Input: part model. Units: mm. Frame: model coordinates. A direction names the side the tool comes from. Coordinates: 2 decimals unless noted, no trailing zeros.
(1) Mould query, pull axis X, two halves, no side actions, for faces 1 (the face through (344, 406, 5)), 2 (the face through (197, 254, 10)). Classes: released by +X, released by -X, zero draft, split by the parting line, or undercut.
(2) Section A-A, the plane z = 2.25. Give the number of separate pieces and of enclosed holes in the cut face, then the cut area to 3 significant figures.
(3) Set-up query: faces 3 (the face through (197, 500, 5)), 4 (the face through (255, 450, 5)), 5 (the face through (369, 414, 5)). Return all of +Z, -Z, +X, -X, +Y, -Y with unobstructed straight access to the full face (end or side cutting, diameter ignored); none if empty.
(4) Line query: L1, parallel to Y at x = 331.75, z = 5.25; L2, parallel to Y at x = 366.5, z = 1; L3, parallel to Y at x = 192.5, z = 3.25. Output: solid intervals per line, ascending.
(5) Contact query for flat-ended pins moving along their axis: P1, Ø5.5, axis at x = 289.5, y = 480, coming from the -Z side; P2, Ø3, axis at y = 362, z = 9, coming from the -X side. Output: stop coordinate, or through.
```python
from build123d import *

# Parameters (mm, degrees)
SKETCH1_W           = 400
SKETCH1_H           = 500
BOSS_EXTRUDE1_DEPTH = 10
CUT_EXTRUDE12_DEPTH = 20
FILLET2_R           = 5
CUT_EXTRUDE16_DEPTH = 32
SKETCH19_R          = 3
SKETCH19_R_2        = 3.35
CUT_EXTRUDE17_DEPTH = 124
CUT_EXTRUDE18_DEPTH = 5


with BuildPart() as part:
    # Sketch1 → Boss-Extrude1 (new body)
    with BuildSketch(Plane.XY):
        with Locations((200, 250)):
            Rectangle(SKETCH1_W, SKETCH1_H)
    extrude(amount=BOSS_EXTRUDE1_DEPTH)

    # Sketch15 → Cut-Extrude12 (cut)
    with BuildSketch(Plane.XY.offset(10)):
        with BuildLine():
            Line((155, 460), (245, 460))
            ThreePointArc((245, 460), (255, 450), (245, 440))
            Line((245, 440), (155, 440))
            ThreePointArc((155, 440), (145, 450), (155, 460))
        make_face()
    extrude(amount=-CUT_EXTRUDE12_DEPTH, mode=Mode.SUBTRACT)

    # Fillet2
    fillet2_edges = [part.edges().sort_by_distance(p)[0] for p in [
        (0, 250, 10),
        (400, 250, 10),
    ]]
    fillet(fillet2_edges, radius=FILLET2_R)

    # Sketch18 → Cut-Extrude16 (cut)
    with BuildSketch(Plane.XY.offset(10)):
        with BuildLine():
            Line((351.5, 399.75), (336.5, 399.75))
            ThreePointArc((336.5, 399.75), (333.75, 402.5), (336.5, 405.25))
            Line((336.5, 405.25), (351.5, 405.25))
            ThreePointArc((351.5, 405.25), (354.25, 402.5), (351.5, 399.75))
        make_face()
        with BuildLine():
            Line((376.5, 407.25), (361.5, 407.25))
            ThreePointArc((361.5, 407.25), (358.75, 410), (361.5, 412.75))
            Line((361.5, 412.75), (376.5, 412.75))
            ThreePointArc((376.5, 412.75), (379.25, 410), (376.5, 407.25))
        make_face()
        with BuildLine():
            Line((376.5, 392.25), (361.5, 392.25))
            ThreePointArc((361.5, 392.25), (358.75, 395), (361.5, 397.75))
            Line((361.5, 397.75), (376.5, 397.75))
            ThreePointArc((376.5, 397.75), (379.25, 395), (376.5, 392.25))
        make_face()
    extrude(amount=-CUT_EXTRUDE16_DEPTH, mode=Mode.SUBTRACT)

    # Sketch19 → Cut-Extrude17 (cut)
    with BuildSketch(Plane(origin=(0, 0, 0), x_dir=(-1, 0, 0), z_dir=(0, 0, -1))):
        with Locations((-380, 145.5)):
            Circle(SKETCH19_R)
        with Locations((-380, 127.5)):
            Circle(SKETCH19_R)
        with Locations((-380, 17)):
            Circle(SKETCH19_R_2)
        with Locations((-17, 17)):
            Circle(SKETCH19_R_2)
        with Locations((-17, 145.5)):
            Circle(SKETCH19_R)
        with Locations((-17, 127.5)):
            Circle(SKETCH19_R)
        with Locations((-113.25, 317.5)):
            Circle(SKETCH19_R)
        with Locations((-113.25, 331.5)):
            Circle(SKETCH19_R)
        with Locations((-151.75, 317.5)):
            Circle(SKETCH19_R)
        with Locations((-151.75, 331.5)):
            Circle(SKETCH19_R)
        with Locations((-293.25, 317.5)):
            Circle(SKETCH19_R)
        with Locations((-293.25, 331.5)):
            Circle(SKETCH19_R)
        with Locations((-331.75, 317.5)):
            Circle(SKETCH19_R)
        with Locations((-331.75, 331.5)):
            Circle(SKETCH19_R)
        with Locations((-17, 336)):
            Circle(SKETCH19_R)
        with Locations((-17, 351)):
            Circle(SKETCH19_R)
        with Locations((-17, 480)):
            Circle(SKETCH19_R_2)
        with Locations((-109.5, 480)):
            Circle(SKETCH19_R)
        with Locations((-127.5, 480)):
            Circle(SKETCH19_R)
        with Locations((-271.5, 480)):
            Circle(SKETCH19_R)
        with Locations((-289.5, 480)):
            Circle(SKETCH19_R)
        with Locations((-380, 480)):
            Circle(SKETCH19_R_2)
        with Locations((-382.5, 353.25)):
            Circle(SKETCH19_R)
        with Locations((-382.5, 368.25)):
            Circle(SKETCH19_R)
        with Locations((-51.5, 323)):
            Circle(SKETCH19_R_2)
        with Locations((-51.5, 17)):
            Circle(SKETCH19_R_2)
    extrude(amount=-CUT_EXTRUDE17_DEPTH, mode=Mode.SUBTRACT)

    # Sketch18<4> → Cut-Extrude18 (cut)
    # profile 1 of 3: a face of its own
    with BuildSketch(Plane.XY.offset(10)):
        with BuildLine():
            Line((351.5, 397), (336.5, 397))
            ThreePointArc((336.5, 397), (331, 402.5), (336.5, 408))
            Line((336.5, 408), (351.5, 408))
            ThreePointArc((351.5, 408), (357, 402.5), (351.5, 397))
        make_face()
        with BuildLine():
            Line((351.5, 399.75), (336.5, 399.75))
            ThreePointArc((336.5, 399.75), (333.75, 402.5), (336.5, 405.25))
            Line((336.5, 405.25), (351.5, 405.25))
            ThreePointArc((351.5, 405.25), (354.25, 402.5), (351.5, 399.75))
        make_face(mode=Mode.SUBTRACT)
    # profile 2 of 3: a face of its own
    with BuildSketch(Plane.XY.offset(10)):
        with BuildLine():
            Line((376.5, 404.5), (361.5, 404.5))
            ThreePointArc((361.5, 404.5), (356, 410), (361.5, 415.5))
            Line((361.5, 415.5), (376.5, 415.5))
            ThreePointArc((376.5, 415.5), (382, 410), (376.5, 404.5))
        make_face()
        with BuildLine():
            Line((376.5, 407.25), (361.5, 407.25))
            ThreePointArc((361.5, 407.25), (358.75, 410), (361.5, 412.75))
            Line((361.5, 412.75), (376.5, 412.75))
            ThreePointArc((376.5, 412.75), (379.25, 410), (376.5, 407.25))
        make_face(mode=Mode.SUBTRACT)
    # profile 3 of 3: a face of its own
    with BuildSketch(Plane.XY.offset(10)):
        with BuildLine():
            Line((376.5, 389.5), (361.5, 389.5))
            ThreePointArc((361.5, 389.5), (356, 395), (361.5, 400.5))
            Line((361.5, 400.5), (376.5, 400.5))
            ThreePointArc((376.5, 400.5), (382, 395), (376.5, 389.5))
        make_face()
        with BuildLine():
            Line((376.5, 392.25), (361.5, 392.25))
            ThreePointArc((361.5, 392.25), (358.75, 395), (361.5, 397.75))
            Line((361.5, 397.75), (376.5, 397.75))
            ThreePointArc((376.5, 397.75), (379.25, 395), (376.5, 392.25))
        make_face(mode=Mode.SUBTRACT)
    extrude(amount=-CUT_EXTRUDE18_DEPTH, mode=Mode.SUBTRACT)


solid = part.part
```
Report:
1. face 1: undercut
1. face 2: zero draft
2. separate pieces: 1
2. enclosed holes: 30
2. area: 197,000 mm2
3. face 3: +Z, -Z, +X, -X, +Y
3. face 4: +Z, -Z
3. face 5: +Z
4. L1: y = 0 to 314.5, 320.5 to 328.5, 334.5 to 399.73, 405.27 to 500
4. L2: y = 0 to 392.25, 397.75 to 407.25, 412.75 to 500
4. L3: y = 0 to 440, 460 to 500
5. P1: passes through
5. P2: stops at x = 0.67
